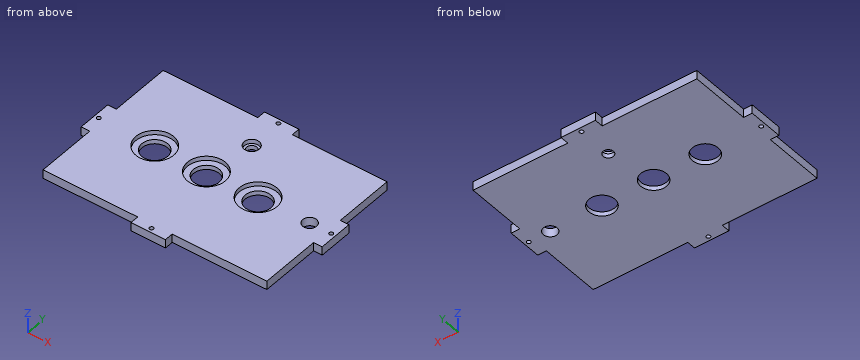
from build123d import *

# Parameters (mm, degrees)
F0_R     = 1.4605
F0_R_2   = 13.97
F0_R_3   = 5.08
F0_R_4   = 5.588
F1_DEPTH = 6.35
F0_R_5   = 9.525
F2_DEPTH = 3.175
F0_R_6   = 3.81
F3_DEPTH = 3.175


with BuildPart() as f1:
    # F0 (on Top) → F1 (new body)
    with BuildSketch(Plane.XY):
        Polygon((-12.7, -63.5), (12.7, -63.5), (12.7, -57.149999), (82.549999, -57.149999), (82.549999, -12.7), (88.9, -12.7), (88.9, 12.7), (82.549999, 12.7), (82.549999, 57.149999), (12.7, 57.149999), (12.7, 63.5), (-12.7, 63.5), (-12.7, 57.149999), (-82.549999, 57.149999), (-82.549999, 12.7), (-88.9, 12.7), (-88.9, -12.7), (-82.549999, -12.7), (-82.549999, -57.149999), (-12.7, -57.149999), align=None)
        with Locations((0, -60.324999)):
            Circle(F0_R, mode=Mode.SUBTRACT)
        with Locations((-85.724999, 0)):
            Circle(F0_R, mode=Mode.SUBTRACT)
        with Locations((-44.45, 0)):
            Circle(F0_R_2, mode=Mode.SUBTRACT)
        with Locations((-6.35, 0)):
            Circle(F0_R_2, mode=Mode.SUBTRACT)
        with Locations((31.75, 0)):
            Circle(F0_R_2, mode=Mode.SUBTRACT)
        with Locations((69.849998, 0)):
            Circle(F0_R_3, mode=Mode.SUBTRACT)
        with Locations((85.724999, 0)):
            Circle(F0_R, mode=Mode.SUBTRACT)
        with Locations((0, 34.924999)):
            Circle(F0_R_4, mode=Mode.SUBTRACT)
        with Locations((0, 60.324999)):
            Circle(F0_R, mode=Mode.SUBTRACT)
    extrude(amount=F1_DEPTH)

    # F0 (on Top) → F2 (join)
    with BuildSketch(Plane.XY):
        with Locations((-44.45, 0)):
            Circle(F0_R_2)
        with Locations((-44.45, 0)):
            Circle(F0_R_5, mode=Mode.SUBTRACT)
        with Locations((-6.35, 0)):
            Circle(F0_R_2)
        with Locations((-6.35, 0)):
            Circle(F0_R_5, mode=Mode.SUBTRACT)
        with Locations((31.75, 0)):
            Circle(F0_R_2)
        with Locations((31.75, 0)):
            Circle(F0_R_5, mode=Mode.SUBTRACT)
    extrude(amount=F2_DEPTH)

    # F0 (on Top) → F3 (join)
    with BuildSketch(Plane.XY):
        with Locations((0, 34.924999)):
            Circle(F0_R_4)
        with Locations((0, 34.924999)):
            Circle(F0_R_6, mode=Mode.SUBTRACT)
    extrude(amount=F3_DEPTH)


solid = f1.part
Read the model definition and answer for the solid it produces. Units are mm, in the model's axes. Give positions to 0.01 mm unless a question says otherwise; leave off trailing zeros. Write each loop counter-clockwise with the first axis right and the second up, starting at its lowest first coordinate (ties: lowest second). Pieces come first, ordered by that corner, then holes. Notation, with made-up numbers: (34, 66.5) -> (77, 66.5) arc R15 ccw to (77, 89.5) -> close; hole circle Ø7 at (72, 44). An arc over 180 degrees is marked (long way). Answer as a JSON object with one key per item and string values. Group by question number.
1) Find section B-B (z = 1.25). Count the separate pieces of the cut face and the enclosed holes in it, and give its area (3 significant figures).
2) Find section C-C (y = -24). Write down the section's boundary in (x, z).
3) Consider L1, parallel to X at y = 58.5, z = 1; L2, parallel to X at y = -36.5, z = 4.5; L3, parallel to Y at x = -6.35, z = 5.3. Determine where each line is inside the solid, lowest interval first. Write a range as from..to.
4) Find section A-A (x = -44.45). Write down the section's boundary in (y, z) (3 decimals), and give its area (3 significant figures).
5) Each of these flat-tipped pins is pushed along its axis until it touches: P1, Ø1.5, axis at y = 37, z = 4.5, coming from the +X side; P2, Ø2.5, axis at x = -85.725, y = 0, coming from the +Z side; P3, Ø3, axis at x = -48.5, z = 4.5, coming from the +Y side; P4, Ø1.9, axis at y = 32.5, z = 2, coming from the -X side. Where does it stop, or does it pass through?
Values follow:
{
 "1": {"separate pieces": "1", "enclosed holes": "9", "area": "18,500 mm2"},
 "2": {"outline": "(-82.55, 0) -> (82.55, 0) -> (82.55, 6.35) -> (-82.55, 6.35) -> close"},
 "3": {"L1": "x = -12.7..12.7", "L2": "x = -82.55..82.55", "L3": "y = -63.5..-13.97, 13.97..63.5"},
 "4": {"outline": "(-57.15, 0) -> (-9.525, 0) -> (-9.525, 3.175) -> (-13.97, 3.175) -> (-13.97, 6.35) -> (-57.15, 6.35) -> close; (9.525, 0) -> (57.15, 0) -> (57.15, 6.35) -> (13.97, 6.35) -> (13.97, 3.175) -> (9.525, 3.175) -> close", "area": "577 mm2"},
 "5": {"P1": "stops at x = 82.55", "P2": "passes through", "P3": "stops at y = 57.15", "P4": "stops at x = -82.55"}
}
